The model under review builds one solid part; all positions refer to its coordinate system, in mm. A direction names the side the tool comes from. Round coordinates to 2 decimals unless told otherwise and drop trailing zeros. Write each loop counter-clockwise with the first axis right and the second up, starting at its lowest first coordinate (ties: lowest second). Pieces come first, ordered by that corner, then holes. Notation, with made-up numbers: (84.25, 9.25) - (128.25, 9.25) arc R5 ccw to (128.25, 16.25) - close; hole circle Ø3 at (59.25, 35.25). An arc over 180 degrees is marked (long way). Write each question's results on one line, items separated by ' | '.
```python
from build123d import *

# Parameters (mm, degrees)
SKETCH4_R           = 40
SKETCH4_R_2         = 5.5
BOSS_EXTRUDE1_DEPTH = 15.875
SKETCH5_R           = 5.5
CUT_EXTRUDE2_DEPTH  = 265.729718277
FILLET1_R           = 10
FILLET2_R           = 20
FILLET3_R           = 10
CUT_EXTRUDE3_DEPTH  = 3.175


with BuildPart() as part:
    # Sketch4 → Boss-Extrude1 (new body)
    with BuildSketch(Plane.XY):
        with BuildLine():
            Line((-142.633865887, -146.080164327), (21.544941406, -195.965223983))
            ThreePointArc((21.544941406, -195.965223983), (33.862932788, -192.99616638), (37.258075063, -180.78874144))
            Line((37.258075063, -180.78874144), (-7.649527095, -12.138772571))
            ThreePointArc((-7.649527095, -12.138772571), (-14.239674224, -4.124786339), (-24.611636772, -3.848367419))
            Line((-24.611636772, -3.848367419), (-147.429933804, -55.967315581))
            ThreePointArc((-147.429933804, -55.967315581), (-176.611366682, -102.704491033), (-142.633865887, -146.080164327))
        make_face()
        with Locations((-128.679206861, -100.153402069)):
            Circle(SKETCH4_R, mode=Mode.SUBTRACT)
        with Locations((25.178967194, -184.005129645)):
            Circle(SKETCH4_R_2, mode=Mode.SUBTRACT)
        with Locations((-19.728634964, -15.355160776)):
            Circle(SKETCH4_R_2, mode=Mode.SUBTRACT)
    extrude(amount=BOSS_EXTRUDE1_DEPTH)

    # Sketch5 → Cut-Extrude2 (cut, through all)
    # profile 1 of 3: a face of its own
    with BuildSketch(Plane.XY.offset(15.875)):
        with BuildLine():
            ThreePointArc((-147.429933804, -55.967315581), (-139.051950222, -53.287570217), (-130.325634952, -52.181647103))
            Line((-130.325634952, -52.181647103), (-81.364667563, -50.50126847))
            ThreePointArc((-81.364667563, -50.50126847), (-71.071592766, -55.316332604), (-68.930846466, -66.476504497))
            Line((-68.930846466, -66.476504497), (-73.912035736, -83.647480421))
            Line((-73.912035736, -83.647480421), (33.260347587, -174.468815318))
            ThreePointArc((33.260347587, -174.468815318), (35.742900566, -177.322816295), (37.258075063, -180.78874144))
            Line((37.258075063, -180.78874144), (-7.649527095, -12.138772571))
            ThreePointArc((-7.649527095, -12.138772571), (-14.239674224, -4.124786339), (-24.611636772, -3.848367419))
            Line((-24.611636772, -3.848367419), (-147.429933804, -55.967315581))
        make_face()
        with Locations((-19.728634964, -15.355160776)):
            Circle(SKETCH5_R, mode=Mode.SUBTRACT)
    # profile 2 of 3: a face of its own
    with BuildSketch(Plane.XY.offset(15.875)):
        with BuildLine():
            Line((20.104564205, -172.581450977), (-76.29204815, -91.851773341))
            Line((-76.29204815, -91.851773341), (-82.579761939, -113.52655345))
            ThreePointArc((-82.579761939, -113.52655345), (-94.695070233, -134.05146186), (-115.189187477, -146.218783616))
            Line((-115.189187477, -146.218783616), (12.828423676, -185.932323147))
            ThreePointArc((12.828423676, -185.932323147), (14.203146627, -178.023377153), (20.104564205, -172.581450977))
        make_face()
    # profile 3 of 3: a face of its own
    with BuildSketch(Plane.XY.offset(15.875)):
        with Locations((-80.935910248, -62.993912992)):
            Circle(SKETCH5_R)
    extrude(amount=-CUT_EXTRUDE2_DEPTH, mode=Mode.SUBTRACT)

    # Fillet1
    fillet1_edges = [part.edges().sort_by_distance(p)[0] for p in [
        (-73.912035736, -83.647480421, 7.9375),
        (-115.189187477, -146.218783616, 7.9375),
        (-76.29204815, -91.851773341, 7.9375),
    ]]
    fillet(fillet1_edges, radius=FILLET1_R)

    # Fillet2
    fillet2_edges = [part.edges().sort_by_distance(p)[0] for p in [
        (20.104564205, -172.581450977, 7.9375),
    ]]
    fillet(fillet2_edges, radius=FILLET2_R)

    # Fillet3
    fillet3_edges = [part.edges().sort_by_distance(p)[0] for p in [
        (12.828423676, -185.932323147, 7.9375),
    ]]
    fillet(fillet3_edges, radius=FILLET3_R)

    # Sketch9 → Cut-Extrude3 (cut, symmetric)
    with BuildSketch(Plane.XY.offset(7.9375)):
        Polygon((-61.249571306, -94.378061257), (-111.793381856, -51.545605705), (-96.460931355, -33.452772516), (-45.917120805, -76.285228067), align=None)
    extrude(amount=CUT_EXTRUDE3_DEPTH, both=True, mode=Mode.SUBTRACT)


solid = part.part
```
Q1. We need section C-C (x = -38). State the section outline as (y, z) points (1 decimal), plus the area to 3 significant figures.
Evaluation:
outline: (-177.9, 0) - (-170.2, 0) - (-170.2, 15.9) - (-177.9, 15.9) - close; (-123.9, 0) - (-114.1, 0) - (-114.1, 15.9) - (-123.9, 15.9) - close | area: 279 mm^2
Q2. Insertion check: P1, Ø8, axis at x = -41.5, y = -108, coming from the +Z side (3 decimals); P2, Ø4, axis at x = -14.5, z = 8, coming from the +Y side; P3, Ø5, axis at y = -74.5, z = 9, coming from the -X side; P4, Ø4, axis at y = -69.5, z = 5, coming from the -X side. Each pin has a flat end and moves straight along its axis. Give the tip position at first contact, or say it passes through.
Evaluation:
P1: stops at z = 15.875 | P2: stops at y = -132.3 | P3: stops at x = -170.73 | P4: stops at x = -167.19
Q3. The part is to be moulded in two halves that separate along Y. For faces 1 (the cylindrical face through (-75.69, -61.34, 13.53)), 2 (the flat face through (-90, -61, 4.762)), 3 (the flat face through (-70.496, -71.873, 2.415)), 4 (the flat face through (-61.694, -170.673, 7.826)), say which applies: released by +Y, released by -Y, zero draft, split by the parting line, or undercut.
Evaluation:
face 1: undercut | face 2: zero draft | face 3: undercut | face 4: released by -Y
Q4. We need section B-B (y = -81). State the section outline as (x, z) points (1 decimal), plus the area to 3 significant figures.
Evaluation:
outline: (-172.7, 0) - (-163.8, 0) - (-163.8, 15.9) - (-172.7, 15.9) - close; (-93.6, 0) - (-72.5, 0) - (-72.5, 4.8) - (-77, 4.8) - (-77, 11.1) - (-72.5, 11.1) - (-72.5, 15.9) - (-93.6, 15.9) - close | area: 447 mm^2
Q5. We need section A-A (y = -118). State the section outline as (x, z) points (3 decimals), plus the area to 3 significant figures.
Evaluation:
outline: (-173.238, 0) - (-164.477, 0) - (-164.477, 15.875) - (-173.238, 15.875) - close; (-92.881, 0) - (-84.12, 0) - (-84.12, 15.875) - (-92.881, 15.875) - close; (-45.069, 0) - (-33.375, 0) - (-33.375, 15.875) - (-45.069, 15.875) - close | area: 464 mm^2
Q6. Tool access review of faces 5 (the flat face through (-81.557, -110.002, 8.049)), 6 (the flat face through (-70.496, -71.873, 13.527)), 7 (the flat face through (-86, -112, 0)): name each direction out of +Z, -Z, +X, -X, +Y, -Y from which nothing blocks a thin tool from reaching the whole face with its end or side.
Evaluation:
face 5: +Z, -Z | face 6: +Z, -Z, +X | face 7: -Z, +X, -X, +Y, -Y
Q7. We need section D-D (x = -14). State the section outline as (y, z) points (3 decimals), plus the area to 3 significant figures.
Evaluation:
outline: (-185.165, 0) - (-177.61, 0) - (-177.61, 15.875) - (-185.165, 15.875) - close; (-144.02, 0) - (-134.419, 0) - (-134.419, 15.875) - (-144.02, 15.875) - close | area: 272 mm^2
Q8. For probe 1 along X at (y, z) = (-132, 11.5); probe 2 along X at (y, z) = (-127, 7); probe 3 along Y at (x, z) = (-93, 4.25), list the stretches that pass through material, from the lowest coordinate up.
Evaluation:
probe 1: x = -164.59 to -152.88, -104.48 to -92.77, -28.35 to -16.85 | probe 2: x = -168.47 to -158.33, -99.03 to -88.89, -34.32 to -22.75 | probe 3: y = -161.16 to -153.1, -132.26 to -118.24, -82.07 to -50.9
